The listing builds one solid part. Answer for the finished solid, in the listing's coordinates (mm). Face numbers are marked on the shaded views. A direction names the side the tool comes from. Round coordinates to 2 decimals unless told otherwise and drop trailing zeros. Loops run counter-clockwise (first coordinate to the right, second up) from the corner with the lowest first, then second, coordinate; pieces in that order, holes last. Notation, with made-up numbers: (16.25, 77.5) - (65.25, 77.5) arc R19 cw to (65.25, 97.5) - close; hole circle Ø11 at (38, -39). An arc over 180 degrees is marked (long way). One line per item, written item: value.
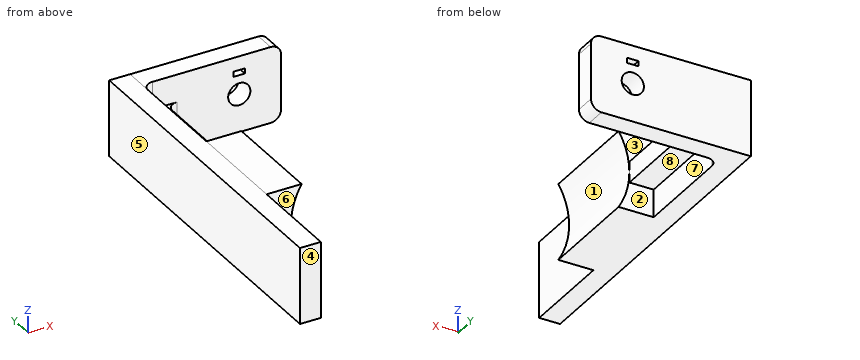
```python
from build123d import *

# Parameters (mm, degrees)
SKETCH2_W           = 6
SKETCH2_H           = 22
BOSS_EXTRUDE2_DEPTH = 95
SKETCH3_R           = 3.2
SKETCH3_W           = 3.2
SKETCH3_H           = 1.5
BOSS_EXTRUDE3_DEPTH = 6
SKETCH4_W           = 6
SKETCH4_H           = 62
BOSS_EXTRUDE4_DEPTH = 7
BOSS_EXTRUDE5_DEPTH = 30
FILLET4_R           = 3


with BuildPart() as part:
    # Sketch2 → Boss-Extrude2 (new body)
    with BuildSketch(Plane(origin=(0, 0, 0), x_dir=(1, 0, 0), z_dir=(0, 1, 0))):
        with Locations((-31, 0)):
            Rectangle(SKETCH2_W, SKETCH2_H)
    extrude(amount=BOSS_EXTRUDE2_DEPTH)

    # Sketch3 → Boss-Extrude3 (add)
    with BuildSketch(Plane(origin=(0, 95, 0), x_dir=(1, 0, 0), z_dir=(0, 1, 0))):
        with BuildLine():
            Line((-28, 11), (9.041317524, 11))
            ThreePointArc((9.041317524, 11), (11.162637868, 10.121320344), (12.041317524, 8))
            Line((12.041317524, 8), (12.041317524, -7.97837003))
            ThreePointArc((12.041317524, -7.97837003), (11.162637868, -10.099690374), (9.041317524, -10.97837003))
            Line((9.041317524, -10.97837003), (-28, -10.97837003))
            Line((-28, -10.97837003), (-28, 11))
        make_face()
        with Locations(Location((0, 0, 0), (0, 0, 270))):
            Circle(SKETCH3_R, mode=Mode.SUBTRACT)
        with Locations((0, -6.25)):
            Rectangle(SKETCH3_W, SKETCH3_H, mode=Mode.SUBTRACT)
    extrude(amount=-BOSS_EXTRUDE3_DEPTH)

    # Sketch4 → Boss-Extrude4 (add)
    with BuildSketch(Plane(origin=(-28, 0, 0), x_dir=(0, 0, -1), z_dir=(1, 0, 0))):
        with Locations((0.010814985, 58)):
            Rectangle(SKETCH4_W, SKETCH4_H)
    extrude(amount=BOSS_EXTRUDE4_DEPTH)

    # Sketch5 → Boss-Extrude5 (add)
    with BuildSketch(Plane.XZ.offset(-27)):
        with BuildLine():
            Line((-28, 10.97837003), (-17.901826484, 10.97837003))
            ThreePointArc((-17.901826484, 10.97837003), (-20.999996165, -0.012691382), (-17.88854382, -11))
            Line((-17.88854382, -11), (-28, -11))
            Line((-28, -11), (-28, 10.97837003))
        make_face()
    extrude(amount=-BOSS_EXTRUDE5_DEPTH)

    # Fillet4
    fillet4_edges = [part.edges().sort_by_distance(p)[0] for p in [
        (-28, 89, -7.005407492),
        (-28, 89, 6.983777523),
        (-21, 89, -0.010814985),
    ]]
    fillet(fillet4_edges, radius=FILLET4_R)


solid = part.part
```
1) Consider L1, parallel to X at y = 92.6, z = 0; L2, parallel to X at y = 58, z = 9.75; L3, parallel to Y at x = -17.5, z = 2.75. Determine where each line is inside the solid, lowest interval first.
Final values:
L1: -34 to -3.2, 3.2 to 12.04
L2: -34 to -28
L3: 89 to 95
2) For a pull along Y with two mould halves and no side action, classify the marked faces 5, 6, 7 and 8 as released by +Y, released by -Y, zero draft, split by the parting line, or undercut.
Final values:
face 5: zero draft
face 6: released by -Y
face 7: undercut
face 8: undercut
3) A cutting plane is placed at A-A on x = 0. Give the vertices of the cut face in (y, z), and give its area (3 significant figures).
Final values:
outline: (89, -11) - (95, -11) - (95, -3.2) - (89, -3.2) - close; (89, 3.2) - (95, 3.2) - (95, 5.5) - (89, 5.5) - close; (89, 7) - (95, 7) - (95, 10.98) - (89, 10.98) - close
area: 84.5 mm2
4) A cutting plane is placed at D-D on x = -19.5. Give the vertices of the cut face in (y, z), and give its area (3 significant figures).
Final values:
outline: (27, -11) - (57, -11) - (57, -7.79) - (27, -7.79) - close; (27, 7.79) - (57, 7.79) - (57, 10.98) - (27, 10.98) - close; (88.6, -3.01) - (89, -3.01) - (89, -11) - (95, -11) - (95, 10.98) - (89, 10.98) - (89, 2.99) - (88.6, 2.99) - close
area: 326 mm2
5) A cutting plane is placed at C-C on z = -7. Give the vertices of the cut face in (x, y), and give its area (3 significant figures).
Final values:
outline: (-34, 0) - (-28, 0) - (-28, 27) - (-19.8, 27) - (-19.8, 57) - (-28, 57) - (-28, 86) arc R3 cw to (-25, 89) - (12.04, 89) - (12.04, 95) - (-34, 95) - close
area: 1,060 mm2
6) For the marked faces 1, 2, 3 and 4, determine the directions among +Z, -Z, +X, -X, +Y, -Y from which every point of the face is accessible in a straight line to the end or side of a thin tool.
Final values:
face 1: +X, -Y
face 2: -Z, +X
face 3: +Z, +X
face 4: +Z, -Z, +X, -X, -Y
7) Each of these flat-tipped pins is pushed along its axis until it touches: pin 1 Ø5 at (x, y) = (-25, 67) entering from -Z; pin 2 Ø8 at (x, y) = (-23.5, 41) entering from +Z; pin 3 Ø3 at (x, y) = (-25.5, 70) entering from +Z. Where does it stop, or does it pass through?
Final values:
pin 1: z = -3.01
pin 2: z = 10.98
pin 3: z = 2.99
